from build123d import *

# Parameters (mm, degrees)
SKETCH1_W           = 70
SKETCH1_H           = 70
BOSS_EXTRUDE1_DEPTH = 3.175
SKETCH2_W           = 1
SKETCH2_H           = 16.56370183
CUT_EXTRUDE1_DEPTH  = 3.175
SKETCH3_W           = 30
SKETCH3_H           = 5
SKETCH3_W_2         = 5
SKETCH3_H_2         = 30
CUT_EXTRUDE2_DEPTH  = 10


with BuildPart() as part:
    # Sketch1 → Boss-Extrude1 (new body)
    with BuildSketch(Plane(origin=(0, 0, 0), x_dir=(1, 0, 0), z_dir=(0, 1, 0))):
        Rectangle(SKETCH1_W, SKETCH1_H)
    extrude(amount=BOSS_EXTRUDE1_DEPTH)

    # Sketch2 → Cut-Extrude1 (cut)
    with BuildSketch(Plane(origin=(0, 3.175, 0), x_dir=(1, 0, 0), z_dir=(0, 1, 0))):
        with Locations((0.5, 26.718149085)):
            Rectangle(SKETCH2_W, SKETCH2_H)
    extrude(amount=-CUT_EXTRUDE1_DEPTH, mode=Mode.SUBTRACT)

    # Sketch3 → Cut-Extrude2 (cut)
    with BuildSketch(Plane(origin=(0, 3.175, 0), x_dir=(1, 0, 0), z_dir=(0, 1, 0))):
        with Locations((10, -32.5)):
            Rectangle(SKETCH3_W, SKETCH3_H)
        with Locations((32.5, -15)):
            Rectangle(SKETCH3_W_2, SKETCH3_H_2)
        with Locations((32.5, 32.5)):
            Rectangle(SKETCH3_W_2, SKETCH3_H)
    extrude(amount=-CUT_EXTRUDE2_DEPTH, mode=Mode.SUBTRACT)


solid = part.part
Verification items for the finished model (mm, model axes). A direction names the side the tool comes from. Give positions to 0.01 mm unless a question says otherwise; leave off trailing zeros. Loops run counter-clockwise (first coordinate to the right, second up) from the corner with the lowest first, then second, coordinate; pieces in that order, holes last.
1) Set-up check for faces 1 (the flat face through (-18, 2, -35)), 2 (the flat face through (32, 2, 0)), 3 (the flat face through (30, 2, -32)), 4 (the flat face through (10, 2, 30)), 5 (the flat face through (1, 2, -27)): record each of +Z, -Z, +X, -X, +Y, -Y from which the full face is reachable in a straight line by a thin tool's end or side.
2) Sectioned sample at B-B, the plane z = 12.5. Enter the section's corners in (x, y) (3 decimals), then the cut area to 3 significant figures.
3) Thickness scan on line 1 along X through (y, z) = (2.6, -23.5); line 2 along Z through (x, y) = (24.5, 0.4). Record the ranges inside material, lowest first.
4) Draft check along Z on faces 6 (the flat face through (35, 2, 33)), 7 (the flat face through (30, 2, 35)), 8 (the flat face through (32, 2, 30)), 9 (the flat face through (30, 2, 15)). Enter one of: pulls with the +Z half, pulls with the -Z half, needs draft (parallel to the pull), parting line crosses it, or undercut.
5) Depth check by flat-ended pin: pin 1 Ø0.5 at (x, y) = (0.5, 1.5) entering from -Z; pin 2 Ø1.6 at (y, z) = (1.5, -33.5) entering from +X; pin 3 Ø1 at (x, y) = (33, 2) entering from -Z. Enter the tip coordinate at first touch or a pass-through.
6) Sectioned sample at C-C, the plane x = 16. Enter the section's corners in (y, z) (3 decimals), then the cut area to 3 significant figures.
7) Sectioned sample at A-A, the plane y = 2.1. Enter the section's corners in (x, z).
Answers:
1. face 1: -Z, +X, -X, +Y, -Y
1. face 2: +X, +Y, -Y
1. face 3: -Z, +X, +Y, -Y
1. face 4: +Z, +Y, -Y
1. face 5: -Z, +Y, -Y
2. outline: (-35, 0) - (30, 0) - (30, 3.175) - (-35, 3.175) - close
2. area: 206 mm2
3. line 1: x = -35 to 0, 1 to 35
3. line 2: z = -35 to 30
4. face 6: needs draft
4. face 7: pulls with the +Z half
4. face 8: undercut
4. face 9: undercut
5. pin 1: stops at z = -18.44
5. pin 2: stops at x = 30
5. pin 3: stops at z = -30
6. outline: (0, -35) - (3.175, -35) - (3.175, 30) - (0, 30) - close
6. area: 206 mm2
7. outline: (-35, -35) - (0, -35) - (0, -18.44) - (1, -18.44) - (1, -35) - (30, -35) - (30, -30) - (35, -30) - (35, 0) - (30, 0) - (30, 30) - (35, 30) - (35, 35) - (25, 35) - (25, 30) - (-5, 30) - (-5, 35) - (-35, 35) - close
